from build123d import *

# Parameters (mm, degrees)
F0_W     = 120
F0_H     = 120
F1_DEPTH = 30
F2_R     = 35.3192378902
F3_DEPTH = 20
F4_R     = 25.158067948
F5_DEPTH = 106.934
F6_R     = 5
F7_R     = 1.5
F8_T     = -3


with BuildPart() as f1:
    # F0 (on Front) → F1 (new body)
    with BuildSketch(Plane.XZ):
        with Locations((29.2758518457, -4.3157362938)):
            Rectangle(F0_W, F0_H)
    extrude(amount=F1_DEPTH)

    # F2 (on face) → F3 (join)
    with BuildSketch(Plane.XZ.offset(30)):
        with Locations((29.2758518457, 0)):
            Circle(F2_R)
    extrude(amount=F3_DEPTH)

    # F4 (on face) → F5 (cut)
    with BuildSketch(Plane.XZ.offset(50)):
        with Locations((29.2758518457, 0)):
            Circle(F4_R)
    extrude(amount=-F5_DEPTH, mode=Mode.SUBTRACT)

    # F6
    f6_edges = [f1.edges().sort_by_distance(p)[0] for p in [
        (29.275852, -30, -64.315736),
        (-30.724148, -30, -4.315736),
        (89.275852, -30, -4.315736),
        (29.275852, -30, 55.684264),
        (-6.043386, -30, 0),
        (-30.724148, -15, 55.684264),
        (89.275852, -15, 55.684264),
        (89.275852, -15, -64.315736),
        (-30.724148, -15, -64.315736),
    ]]
    fillet(f6_edges, radius=F6_R)

    # F7
    f7_edges = [f1.edges().sort_by_distance(p)[0] for p in [
        (-6.043386, -50, 0),
    ]]
    fillet(f7_edges, radius=F7_R)

    # F8
    f8_openings = [f1.faces().sort_by_distance(p)[0] for p in [
        (29.275852, 0, -62.61868),
    ]]
    offset(amount=F8_T, openings=f8_openings)


solid = f1.part
Check sheet for the modelled part. Datum: model origin and axes. Units: mm. A direction names the side the tool comes from. Round coordinates to 2 decimals unless told otherwise and drop trailing zeros. Order: outer loops, then holes, each group sorted by start corner. A loop starts at its lowest first (then second) coordinate and runs counter-clockwise, first axis right, second up.
(1) Scan lines: probe 1 along X at (y, z) = (-45.5, 26); probe 2 along X at (y, z) = (-9.5, 42.5); probe 3 along Z at (x, y) = (16, -22). Record each from-to range of solid material in increasing order.
(2) Cross-section at D-D, the plane y = -33. Enter the section's corners in (x, z), and give its area (3 significant figures).
(3) Go/stop test with flat-tipped pins: P1, Ø2, axis at x = -12.5, z = -8, coming from the -Y side; P2, Ø1, axis at y = -36, z = -13, coming from the +X side; P3, Ø1, axis at x = 46, y = -28.5, coming from the -Z side; P4, Ø12, axis at x = 45, z = -3.5, coming from the +Y side. Record where each tip stops, or that it passes through.
(4) Cross-section at C-C, the plane z = -50. Enter the section's corners in (x, y).
(5) Cross-section at A-A, the plane y = -23. Enter the section's corners in (x, z).
(6) Draft check along Z on faces 4 (the cylindrical face through (3.63, -40.92, -19.67)), 5 (the flat face through (-30.724, -12, -5)), 6 (the cylindrical face through (-29.3, -12.68, -62.81)), 7 (the cylindrical face through (1.145, -23.829, 1.238)). Enter one of: pulls with the +Z half, pulls with the -Z half, needs draft (parallel to the pull), parting line crosses it, or undercut.
(7) Access from +Z, -Z, +X, -X, +Y, -Y to the whole of each face (thin tool, end or side, straight path). Record for faces 1 (the flat face through (16, -30, -40)), 2 (the flat face through (89.276, -12, -5)), 3 (the flat face through (86.276, -12, -5)).
Check sheet entries:
1. probe 1: x = 5.37 to 10.08, 18.46 to 40.09, 48.47 to 53.18
1. probe 2: x = -30.72 to -27.72, 86.28 to 89.28
1. probe 3: z = -64.32 to -61.32, -24.83 to -21.37, 21.37 to 24.83, 52.68 to 55.68
2. outline: circle Ø71.47 at (29.28, 0); circle Ø56.32 at (29.28, 0); hole circle Ø65.15 at (29.28, 0); hole circle Ø50.32 at (29.28, 0)
2. area: 1,180 mm2
3. P1: stops at y = -30
3. P2: stops at x = 62.31
3. P3: stops at z = -63.32
3. P4: passes through
4. outline: (-30.72, -25) arc R5 ccw to (-25.72, -30) - (84.28, -30) arc R5 ccw to (89.28, -25) - (89.28, 0) - (86.28, 0) - (86.28, -25) arc R2 cw to (84.28, -27) - (-25.72, -27) arc R2 cw to (-27.72, -25) - (-27.72, 0) - (-30.72, 0) - close
5. outline: (-30.72, -59.32) arc R5 ccw to (-25.72, -64.32) - (84.28, -64.32) arc R5 ccw to (89.28, -59.32) - (89.28, 50.68) arc R5 ccw to (84.28, 55.68) - (-25.72, 55.68) arc R5 ccw to (-30.72, 50.68) - close; circle Ø56.32 at (29.28, 0); hole (-27.72, -59.32) arc R2 ccw to (-25.72, -61.32) - (84.28, -61.32) arc R2 ccw to (86.28, -59.32) - (86.28, 50.68) arc R2 ccw to (84.28, 52.68) - (-25.72, 52.68) arc R2 ccw to (-27.72, 50.68) - close; hole circle Ø50.32 at (29.28, 0)
6. face 4: undercut
6. face 5: needs draft
6. face 6: pulls with the -Z half
6. face 7: undercut
7. face 1: -Y
7. face 2: +Z, -Z, +X, +Y, -Y
7. face 3: +Y
